Read the model definition and answer for the solid it produces. Units are mm, in the model's axes. A direction names the side the tool comes from. Round coordinates to 2 decimals unless told otherwise and drop trailing zeros. Loops run counter-clockwise (first coordinate to the right, second up) from the corner with the lowest first, then second, coordinate; pieces in that order, holes last. Notation, with made-up numbers: (36, -13.75) - (41, -13.75) arc R29 ccw to (41, 23.25) - close; hole circle Ø6 at (31.25, 68). An arc over 180 degrees is marked (long way). Answer as CSV lines item,"result".
```python
from build123d import *

# Parameters (mm, degrees)
SKETCH2_W           = 40
SKETCH2_H           = 10
BOSS_EXTRUDE1_DEPTH = 40
CUT_EXTRUDE1_START  = -10
CUT_EXTRUDE1_DEPTH  = 10
SKETCH7_R           = 1.782070526
BOSS_EXTRUDE2_DEPTH = 32.5
FILLET2_R           = 1
SKETCH8_W           = 30
SKETCH8_H           = 24
CUT_EXTRUDE2_DEPTH  = 5


# Read off the part's stored shape, not the designer's step: Cut-Extrude1
with BuildPart() as part:
    # Sketch2 → Boss-Extrude1 (new body)
    with BuildSketch(Plane(origin=(0, 0, 0), x_dir=(1, 0, 0), z_dir=(0, 1, 0))):
        Rectangle(SKETCH2_W, SKETCH2_H)
    extrude(amount=BOSS_EXTRUDE1_DEPTH)

    # Cut-Extrude1 outline → Cut-Extrude1 (cut)
    with BuildSketch(Plane(origin=(0, 0, -5), x_dir=(-1, 0, 0), z_dir=(0, 0, -1)).offset(CUT_EXTRUDE1_START)):
        with BuildLine():
            ThreePointArc((-20, 22.360679775), (0, 30), (20, 22.360679775))
            Line((20, 22.360679775), (20, 40))
            Line((20, 40), (-20, 40))
            Line((-20, 40), (-20, 22.360679775))
        make_face()
    extrude(amount=CUT_EXTRUDE1_DEPTH, mode=Mode.SUBTRACT)

    # Sketch7 → Boss-Extrude2 (add)
    with BuildSketch(Plane(origin=(0, 0, 0), x_dir=(1, 0, 0), z_dir=(0, 1, 0))):
        with Locations(Location((0, 0, 0), (0, 0, 90))):
            Circle(SKETCH7_R)
    extrude(amount=BOSS_EXTRUDE2_DEPTH)

    # Fillet2
    fillet2_edges = [part.edges().sort_by_distance(p)[0] for p in [
        (0, 32.5, 1.782070526),
    ]]
    fillet(fillet2_edges, radius=FILLET2_R)

    # Sketch8 → Cut-Extrude2 (cut)
    with BuildSketch(Plane.XY):
        with Locations((0, 12)):
            Rectangle(SKETCH8_W, SKETCH8_H)
    extrude(amount=CUT_EXTRUDE2_DEPTH, mode=Mode.SUBTRACT)


solid = part.part
```
1) A cutting plane is placed at A-A, the plane y = 5.5. Determine the outline of the cut face in (x, z).
Entries:
outline,"(-20, -5) - (20, -5) - (20, 5) - (15, 5) - (15, 0) - (-15, 0) - (-15, 5) - (-20, 5) - close"
2) A cutting plane is placed at D-D, the plane y = 25.5. Determine the outline of the cut face in (x, z).
Entries:
outline,"(-15.8, -5) - (15.8, -5) - (15.8, 5) - (-15.8, 5) - close"
3) The mould has two halves that part along X. Classify faces 1 (the face through (-20, 11, 0)), 2 (the face through (-15, 12, 2)), 3 (the face through (0, 15, -5)), 4 (the face through (0, 30, 2)): pulls with the +X half, pulls with the -X half, needs draft (parallel to the pull), parting line crosses it, or undercut.
Entries:
face 1,"pulls with the -X half"
face 2,"undercut"
face 3,"needs draft"
face 4,"parting line crosses it"
4) A tool of negligible diameter and unlimited length cuts with its end or side. For faces 5 (the face through (-3, 25, 5)), 6 (the face through (1.58, 30.71, -0.82)), 7 (the face through (15, 12, 2)), from which of +Z, -Z, +X, -X, +Y, -Y can it reach the whole face along a straight path? Write none if from no direction.
Entries:
face 5,"+Z, +X, -X, +Y, -Y"
face 6,"+Y"
face 7,"+Z, -Y"
5) A cutting plane is placed at C-C, the plane x = 13. Determine the outline of the cut face in (y, z), plus the area to 3 significant figures.
Entries:
outline,"(0, -5) - (27.04, -5) - (27.04, 5) - (24, 5) - (24, 0) - (0, 0) - close"
area,"150 mm^2"
6) Each of these flat-tipped pins is pushed along its axis until it touches: P1, Ø6, axis at x = 3.5, z = 3.5, coming from the +Y side; P2, Ø7, axis at x = 5.5, y = 11.5, coming from the +Z side; P3, Ø2, axis at y = 27, z = -3, coming from the +X side. Where does it stop, or does it pass through?
Entries:
P1,"stops at y = 30"
P2,"stops at z = 0"
P3,"stops at x = 14.97"
7) A cutting plane is placed at B-B, the plane z = 2.25. Determine the outline of the cut face in (x, y).
Entries:
outline,"(-20, 0) - (-15, 0) - (-15, 24) - (15, 24) - (15, 0) - (20, 0) - (20, 22.36) arc R30 ccw to (-20, 22.36) - close"
8) Find the intervals of material crossed by line 1 (X direction, y = 2.5, z = 4); line 2 (Z direction, x = -13.5, y = 7.5); line 3 (Y direction, x = -0.5, z = 3), in increasing order.
Entries:
line 1,"x = -20 to -15, 15 to 20"
line 2,"z = -5 to 0"
line 3,"y = 24 to 30"
